Check sheet for the modelled part. Datum: model origin and axes. Units: mm. A direction names the side the tool comes from. Round coordinates to 2 decimals unless told otherwise and drop trailing zeros. Write each loop counter-clockwise with the first axis right and the second up, starting at its lowest first coordinate (ties: lowest second). Pieces come first, ordered by that corner, then holes. Notation, with made-up numbers: (-17.75, 71.25) - (17.25, 71.25) arc R14 cw to (17.25, 91.25) - close; hole circle Ø11 at (20, 41). An arc over 180 degrees is marked (long way). Answer as a JSON object with one key per item and string values. Group by question number.
Item 1: Sectioned sample at C-C on y = 8.5. Record the boundary of the cut face in (x, z), plus the area to 3 significant figures.
Item 2: Gauge pin test, flat ends, axial feed: P1, Ø1.5, axis at y = 24, z = 3.5, coming from the +X side; P2, Ø6, axis at y = 25, z = 0.5, coming from the -X side; P3, Ø2, axis at x = 1, y = 28, coming from the -Z side; P4, Ø1.5, axis at x = -3.5, y = 24.5, coming from the -Z side. Record the tip position at first contact, or that the pin passes through.
Item 3: Sectioned sample at A-A on z = 0. Record the boundary of the cut face in (x, y).
Item 4: Set-up check for faces 1 (the flat face through (-2, 38.6, 0)), 2 (the flat face through (-2, 18.6, 3)): record each of +Z, -Z, +X, -X, +Y, -Y from which the full face is reachable in a straight line by a thin tool's end or side.
Item 5: Sectioned sample at B-B on y = 20.5. Record the boundary of the cut face in (x, z), plus the area to 3 significant figures.
Item 6: Thickness scan on line 1 (Y direction, x = 0.75, z = -0.75); line 2 (Z direction, x = -2.25, y = 24.5); line 3 (X direction, y = 9, z = -2). Record the ranges inside material, lowest first.
```python
from build123d import *

# Parameters (mm, degrees)
ESBO_O1_R                = 7.5
RESSALTO_EXTRUS_O1_DEPTH = 18.6
ESBO_O2_R                = 2.5
RESSALTO_EXTRUS_O2_DEPTH = 20
FILETE1_R                = 1


with BuildPart() as part:
    # Esboço1 → Ressalto-extrusão1 (new body)
    with BuildSketch(Plane(origin=(0, 0, 0), x_dir=(1, 0, 0), z_dir=(0, 1, 0))):
        with Locations(Location((-2.131243559, 0, 0), (0, 0, 270))):
            Circle(ESBO_O1_R)
    extrude(amount=RESSALTO_EXTRUS_O1_DEPTH)

    # Esboço2 → Ressalto-extrusão2 (add)
    with BuildSketch(Plane(origin=(0, 18.6, 0), x_dir=(1, 0, 0), z_dir=(0, 1, 0))):
        with Locations(Location((-2.131243559, 0, 0), (0, 0, 270))):
            Circle(ESBO_O2_R)
    extrude(amount=RESSALTO_EXTRUS_O2_DEPTH)

    # Filete1
    filete1_edges = [part.edges().sort_by_distance(p)[0] for p in [
        (-2.131243559, 0, -7.5),
        (-2.131243559, 18.6, -7.5),
        (-2.131243559, 38.6, -2.5),
    ]]
    fillet(filete1_edges, radius=FILETE1_R)


solid = part.part
```
Completed:
{
 "1": {"outline": "circle Ø15 at (-2.13, 0)", "area": "177 mm²"},
 "2": {"P1": "through", "P2": "x = -4.63", "P3": "z = -1.31", "P4": "z = -2.42"},
 "3": {"outline": "(-9.63, 1) arc R1 ccw to (-8.63, 0) - (4.37, 0) arc R1 ccw to (5.37, 1) - (5.37, 17.6) arc R1 ccw to (4.37, 18.6) - (0.37, 18.6) - (0.37, 37.6) arc R1 ccw to (-0.63, 38.6) - (-3.63, 38.6) arc R1 ccw to (-4.63, 37.6) - (-4.63, 18.6) - (-8.63, 18.6) arc R1 ccw to (-9.63, 17.6) - close"},
 "4": {"face 1": "+Z, -Z, +X, -X, +Y", "face 2": "+Y"},
 "5": {"outline": "circle Ø5 at (-2.13, 0)", "area": "19.6 mm²"},
 "6": {"line 1": "0 to 18.6", "line 2": "-2.5 to 2.5", "line 3": "-9.36 to 5.1"}
}
